Input: part model. Units: mm. Frame: model coordinates. Face numbers are marked on the shaded views. Give positions to 0.01 mm unless a question says otherwise; leave off trailing zeros. Loops run counter-clockwise (first coordinate to the right, second up) from the corner with the lowest first, then second, coordinate; pieces in that order, holes last. Notation, with made-up numbers: (82.25, 38.5) - (98.25, 38.5) arc R15 cw to (98.25, 67.5) - close; hole circle Ø9 at (36, 61). An arc over 180 degrees is marked (long way). One line per question, with ' | ' between items. Start each with the question number.
from build123d import *

# Parameters (mm, degrees)
F0_R     = 15
F0_R_2   = 2
F1_DEPTH = 7
F2_R     = 2
F3_R     = 2


with BuildPart() as f1:
    # F0 (on Top) → F1 (new body)
    with BuildSketch(Plane.XY):
        Circle(F0_R)
        Circle(F0_R_2, mode=Mode.SUBTRACT)
    extrude(amount=F1_DEPTH)

    # F2
    f2_edges = [f1.edges().sort_by_distance(p)[0] for p in [
        (-15, 0, 7),
    ]]
    fillet(f2_edges, radius=F2_R)

    # F3
    f3_edges = [f1.edges().sort_by_distance(p)[0] for p in [
        (-15, 0, 0),
    ]]
    fillet(f3_edges, radius=F3_R)


solid = f1.part
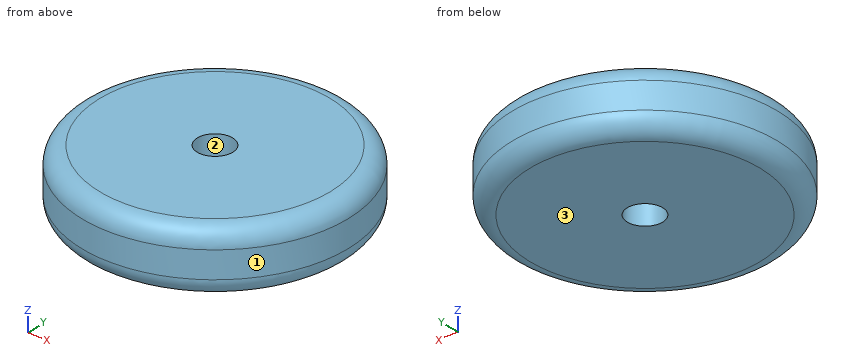
Q1. Section D-D, the plane z = 6. Output: boundary loops of the cut face in (x, y).
Q2. First-contact query: pin 1 (4.5 mm diameter, centred on x = 0, y = 0, fed in from -Z); pin 2 (1 mm diameter, centred on x = -2, z = 3.5, fed in from +Y); pin 3 (4 mm diameter, centred on y = 5, z = 6, fed in from +X); pin 4 (2 mm diameter, centred on x = -1.5, z = 2, fed in from +Y). Flat tips, straight axial feed; report the tip coordinate or a pass-through.
Q3. Section A-A, the plane x = 0. Output: boundary loops of the cut face in (y, z).
Q4. Draft query along X for the marked faces 1, 2 and 3. Return one class per face: +X half, -X half, draft (parallel to the pull), parting line (faces both ways), or undercut.
Q5. Section C-C, the plane z = 2.75. Output: boundary loops of the cut face in (x, y), plus the area to 3 significant figures.
Q6. Line query: L1, parallel to Y at x = 0, z = 3; L2, parallel to Y at x = -7, z = 6; L3, parallel to X at y = -13.5, z = 5.5. Output: solid intervals per line, ascending. Write a range as from..to.
Solved:
1) outline: circle Ø29.46 at (0, 0); hole circle Ø4 at (0, 0)
2) pin 1: stops at z = 0 | pin 2: stops at y = 14.92 | pin 3: stops at x = 14.65 | pin 4: stops at y = 14.99
3) outline: (-15, 2) arc R2 ccw to (-13, 0) - (-2, 0) - (-2, 7) - (-13, 7) arc R2 ccw to (-15, 5) - close; (2, 0) - (13, 0) arc R2 ccw to (15, 2) - (15, 5) arc R2 ccw to (13, 7) - (2, 7) - close
4) face 1: parting line | face 2: undercut | face 3: draft
5) outline: circle Ø30 at (0, 0); hole circle Ø4 at (0, 0) | area: 694 mm²
6) L1: y = -15..-2, 2..15 | L2: y = -12.96..12.96 | L3: x = -6.39..6.39
